Here's how the part is built. I have some questions about the finished solid (model axes, mm). Face numbers are marked on the shaded views. A direction names the side the tool comes from. Coordinates: 2 decimals unless noted, no trailing zeros. Order: outer loops, then holes, each group sorted by start corner. A loop starts at its lowest first (then second) coordinate and runs counter-clockwise, first axis right, second up. Notation, with made-up numbers: (75, 20.5) - (109, 20.5) arc R23 cw to (109, 41.5) - close; hole circle Ø1 at (6.5, 37.25). An arc over 180 degrees is marked (long way). Answer in a Markdown table with one row per item. Add a question column.
Item 1: I want a section at A-A (x = 20). Please give me the cut outline in (y, z) (3 decimals).
Item 2: Will these pins go through, and if not, where does the flat tip stop? pin 1 Ø3 at (x, z) = (16.5, 3) entering from +Y; pin 2 Ø2.5 at (x, y) = (-4, 17.3) entering from -Z; pin 3 Ø4.5 at (y, z) = (14.5, -20) entering from +X; pin 4 Ø1.5 at (x, z) = (-11, -3.5) entering from +Y.
Item 3: If I drill on line 1 along Z through (x, y) = (-0.5, -17); line 2 along X through (y, z) = (-12, -8.5); line 3 along Y through (x, z) = (4.5, -8), over which ranges is the centre line in solid material (lowest first)? Write a range as from..to.
Item 4: Thinking about a two-plate mould opening in Z: for the marked faces 4, 5, 6 and 7, which applies, +Z half, -Z half, draft (parallel to the pull), parting line (faces both ways), or undercut?
Item 5: On a 3-axis mill with a long thin cutter (end or side, diameter ignored), from which of +Z, -Z, +X, -X, +Y, -Y can I reach the whole of each face in a straight line? I mean the marked faces 1, 2 and 3. Say none if no direction works.
Item 6: I want a section at B-B (z = -15.25). Please give me the cut outline in (x, y), plus the area to 3 significant figures.
Item 7: I want a section at C-C (y = 17.3). Please give me the cut outline in (x, z) (3 decimals), plus the area to 3 significant figures.
Item 8: I want a section at D-D (y = -6.5). Please give me the cut outline in (x, z).
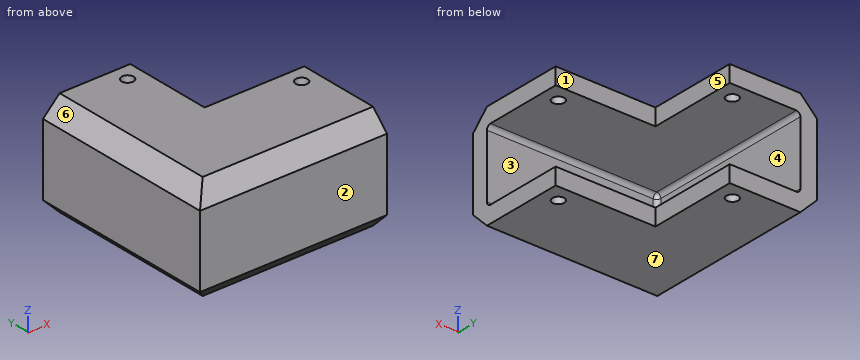
```python
from build123d import *

# Parameters (mm, degrees)
SALIENTE_EXTRUIR1_DEPTH = 4
CROQUIS2_W              = 17.2
CROQUIS2_H              = 41
CROQUIS2_W_2            = 4
SALIENTE_EXTRUIR2_DEPTH = 4
CROQUIS3_W              = 45
CROQUIS3_H              = 21.2
SALIENTE_EXTRUIR3_DEPTH = 4
SALIENTE_EXTRUIR4_DEPTH = 4
REDONDEO1_R             = 1
CHAFL_N1_SIZE           = 4
CROQUIS6_R              = 1.425
CORTAR_EXTRUIR2_DEPTH   = 43.103800304


with BuildPart() as part:
    # Croquis1 → Saliente-Extruir1 (new body)
    with BuildSketch(Plane.XY):
        Polygon((0, 0), (0, 21.3), (-17, 21.3), (-17, -19.7), (24, -19.7), (24, 0), align=None)
    extrude(amount=SALIENTE_EXTRUIR1_DEPTH)

    # Croquis2 → Saliente-Extruir2 (add)
    with BuildSketch(Plane.ZY.offset(17)):
        with Locations((-8.6, 0.8)):
            Rectangle(CROQUIS2_W, CROQUIS2_H)
        with Locations((2, 0.8)):
            Rectangle(CROQUIS2_W_2, CROQUIS2_H)
    extrude(amount=SALIENTE_EXTRUIR2_DEPTH)

    # Croquis3 → Saliente-Extruir3 (add)
    with BuildSketch(Plane.XZ.offset(19.7)):
        with Locations((1.5, -6.6)):
            Rectangle(CROQUIS3_W, CROQUIS3_H)
    extrude(amount=SALIENTE_EXTRUIR3_DEPTH)

    # Croquis4 → Saliente-Extruir4 (add)
    with BuildSketch(Plane(origin=(0, 0, -17.2), x_dir=(-1, 0, 0), z_dir=(0, 0, -1))):
        Polygon((-24, -23.7), (-24, 0), (0, 0), (0, 21.3), (21, 21.3), (21, -23.7), align=None)
    extrude(amount=SALIENTE_EXTRUIR4_DEPTH)

    # Redondeo1
    redondeo1_edges = [part.edges().sort_by_distance(p)[0] for p in [
        (-17, -19.7, -8.6),
        (-17, 0.8, -17.2),
        (3.5, -19.7, -17.2),
        (3.5, -19.7, 0),
        (-17, 0.8, 0),
    ]]
    fillet(redondeo1_edges, radius=REDONDEO1_R)

    # Chaflán1
    chafl_n1_edges = [part.edges().sort_by_distance(p)[0] for p in [
        (-21, -1.2, 4),
        (1.5, -23.7, 4),
        (1.5, -23.7, -21.2),
        (-21, -1.2, -21.2),
    ]]
    chamfer(chafl_n1_edges, length=CHAFL_N1_SIZE)

    # Croquis6 → Cortar-Extruir2 (cut, through all)
    with BuildSketch(Plane(origin=(0, 0, -21.2), x_dir=(-1, 0, 0), z_dir=(0, 0, -1))):
        with Locations(Location((-20, -4, 0), (0, 0, 90))):
            Circle(CROQUIS6_R)
        with Locations(Location((4, 17.3, 0), (0, 0, 90))):
            Circle(CROQUIS6_R)
    extrude(amount=-CORTAR_EXTRUIR2_DEPTH, mode=Mode.SUBTRACT)


solid = part.part
```
Values follow:
| question | item | result |
|---|---|---|
| 1 | outline | (-23.7, -17.2) - (-19.7, -21.2) - (-5.425, -21.2) - (-5.425, -17.2) - (-18.7, -17.2) arc R1 cw to (-19.7, -16.2) - (-19.7, -1) arc R1 cw to (-18.7, 0) - (-5.425, 0) - (-5.425, 4) - (-19.7, 4) - (-23.7, 0) - close; (-2.575, -21.2) - (0, -21.2) - (0, -17.2) - (-2.575, -17.2) - close; (-2.575, 0) - (0, 0) - (0, 4) - (-2.575, 4) - close |
| 2 | pin 1 | stops at y = 0 |
| 2 | pin 2 | passes through |
| 2 | pin 3 | stops at x = 0 |
| 2 | pin 4 | stops at y = -19.7 |
| 3 | line 1 | z = -21.2..-17.2, 0..4 |
| 3 | line 2 | x = -21..-17 |
| 3 | line 3 | y = -23.7..-19.7 |
| 4 | face 4 | undercut |
| 4 | face 5 | draft |
| 4 | face 6 | +Z half |
| 4 | face 7 | -Z half |
| 5 | face 1 | +Z, -Z, +X, +Y |
| 5 | face 2 | +Z, -Z, +X, -X, -Y |
| 5 | face 3 | +X, +Y |
| 6 | outline | (-21, -23.7) - (24, -23.7) - (24, -19.7) - (-16, -19.7) arc R1 cw to (-17, -18.7) - (-17, 21.3) - (-21, 21.3) - close |
| 6 | area | 344 mm^2 |
| 7 | outline | (-21, -17.2) - (-17, -21.2) - (-5.425, -21.2) - (-5.425, -17.2) - (-16, -17.2) arc R1 cw to (-17, -16.2) - (-17, -1) arc R1 cw to (-16, 0) - (-5.425, 0) - (-5.425, 4) - (-17, 4) - (-21, 0) - close; (-2.575, -21.2) - (0, -21.2) - (0, -17.2) - (-2.575, -17.2) - close; (-2.575, 0) - (0, 0) - (0, 4) - (-2.575, 4) - close |
| 7 | area | 198 mm^2 |
| 8 | outline | (-21, -17.2) - (-17, -21.2) - (24, -21.2) - (24, -17.2) - (-16, -17.2) arc R1 cw to (-17, -16.2) - (-17, -1) arc R1 cw to (-16, 0) - (24, 0) - (24, 4) - (-17, 4) - (-21, 0) - close |
